Design review of the part built by this model. Coordinates are the model's own, in mm. A direction names the side the tool comes from. Coordinates: 2 decimals unless noted, no trailing zeros. Order: outer loops, then holes, each group sorted by start corner. A loop starts at its lowest first (then second) coordinate and runs counter-clockwise, first axis right, second up. Notation, with made-up numbers: (33.25, 20) -> (70.25, 20) arc R21 ccw to (70.25, 58) -> close; hole circle Ø10 at (-17.75, 2.25). An arc over 180 degrees is marked (long way). Write item = value, one per line.
```python
from build123d import *

# Parameters (mm, degrees)
F0_W     = 130
F0_H     = 195
F2_DEPTH = 180
F3_START = 150
F1_W     = 139.9999979138
F1_H     = 204.9999979138
F3_DEPTH = 20
F4_T     = -5


with BuildPart() as f2:
    # F0 (on Top) → F2 (new body)
    with BuildSketch(Plane.XY):
        Rectangle(F0_W, F0_H)
    extrude(amount=F2_DEPTH)

    # F1 (on face) → F3 (join)
    with BuildSketch(Plane.XY.offset(F3_START)):
        Rectangle(F1_W, F1_H)
    extrude(amount=F3_DEPTH)

    # F4
    f4_openings = [f2.faces().sort_by_distance(p)[0] for p in [
        (0, 0, 180),
    ]]
    offset(amount=F4_T, openings=f4_openings, kind=Kind.INTERSECTION)


solid = f2.part
```
(1) We need section B-B (x = 50). Write out the cut boundary in (y, z).
Report:
outline = (-102.5, 150) -> (-97.5, 150) -> (-97.5, 0) -> (97.5, 0) -> (97.5, 150) -> (102.5, 150) -> (102.5, 170) -> (97.5, 170) -> (97.5, 180) -> (92.5, 180) -> (92.5, 165) -> (97.5, 165) -> (97.5, 155) -> (92.5, 155) -> (92.5, 5) -> (-92.5, 5) -> (-92.5, 155) -> (-97.5, 155) -> (-97.5, 165) -> (-92.5, 165) -> (-92.5, 180) -> (-97.5, 180) -> (-97.5, 170) -> (-102.5, 170) -> close
(2) For L1, parallel to X at y = 15, z = 162.5; L2, parallel to X at y = -58, z = 80.5; L3, parallel to Z at x = -64, y = 36.5, list the stretches that pass through material, from the lowest coordinate up.
Report:
L1 = -70 to -65, 65 to 70
L2 = -65 to -60, 60 to 65
L3 = 0 to 155, 165 to 180
(3) Insertion check: pin 1 (8 mm diameter, centred on y = 56, z = 107, fed in from +X); pin 2 (3 mm diameter, centred on x = 17, z = 54.5, fed in from -Y); pin 3 (12 mm diameter, centred on x = -36, z = 119.5, fed in from +Y). Each pin has a flat end and moves straight along its axis. Give the tip position at first contact, or say it passes through.
Report:
pin_1 = 65
pin_2 = -97.5
pin_3 = 97.5
(4) The part is to be moulded in two halves that separate along Y. For faces 6 (the flat face through (-1, -92.5, 79)), 7 (the flat face through (-1, -97.5, 74)), 8 (the flat face through (-1, 97.5, 74)), say which applies: released by +Y, released by -Y, zero draft, split by the parting line, or undercut.
Report:
face_6 = undercut
face_7 = released by -Y
face_8 = released by +Y
(5) We need section D-D (z = 111.5). Write out the cut boundary in (x, y).
Report:
outline = (-65, -97.5) -> (65, -97.5) -> (65, 97.5) -> (-65, 97.5) -> close; hole (-60, -92.5) -> (60, -92.5) -> (60, 92.5) -> (-60, 92.5) -> close
(6) We need section A-A (z = 159). Write out the cut boundary in (x, y).
Report:
outline = (-70, -102.5) -> (70, -102.5) -> (70, 102.5) -> (-70, 102.5) -> close; hole (-65, -97.5) -> (65, -97.5) -> (65, 97.5) -> (-65, 97.5) -> close
(7) We need section C-C (y = 40). Write out the cut boundary in (x, z), and give its area (3 significant figures).
Report:
outline = (-70, 150) -> (-65, 150) -> (-65, 0) -> (65, 0) -> (65, 150) -> (70, 150) -> (70, 170) -> (65, 170) -> (65, 180) -> (60, 180) -> (60, 165) -> (65, 165) -> (65, 155) -> (60, 155) -> (60, 5) -> (-60, 5) -> (-60, 155) -> (-65, 155) -> (-65, 165) -> (-60, 165) -> (-60, 180) -> (-65, 180) -> (-65, 170) -> (-70, 170) -> close
area = 2,500 mm²
(8) For faces 1 (the flat face through (-65, -1, 160)), 2 (the flat face through (-65, -1, 74)), 3 (the flat face through (-65, -1, 175)), 4 (the flat face through (65, -1, 74)), 5 (the flat face through (-1, 97.5, 175)), list the 3-axis set-ups (+Z, -Z, +X, -X, +Y, -Y) from which the entire face can be reached by the end or side of a thin tool; tool diameter is ignored.
Report:
face_1 = none
face_2 = -Z, -X, +Y, -Y
face_3 = +Z, -X, +Y, -Y
face_4 = -Z, +X, +Y, -Y
face_5 = +Z, +X, -X, +Y
